Geometry: final body of the model. Coordinates: model frame, mm. A direction names the side the tool comes from. Coordinates: 2 decimals unless noted, no trailing zeros. Write each loop counter-clockwise with the first axis right and the second up, starting at its lowest first coordinate (ties: lowest second). Pieces come first, ordered by that corner, then holes. Notation, with made-up numbers: (88, -33) -> (127, -33) arc R11 cw to (127, -18) -> close; hole circle Ø7 at (82.25, 53). An arc over 180 degrees is marked (long way). One line per item, written item: value.
Autodesk Inventor part; units mm, degrees
ref_plane "YZ Plane" through (0, 0, 0) normal (1, 0, 0) x (0, 1, 0)
ref_plane "XZ Plane" through (0, 0, 0) normal (0, 1, 0) x (-1, 0, 0)
ref_plane "XY Plane" through (0, 0, 0) normal (0, 0, 1) x (1, 0, 0)
sketch "Boceto1" plane through (0, 0, 0) normal (1, 0, 0) x (0, 1, 0)
  line L0 (0, 0) -> (0, 14.3) construction
  line L1 (0, 14.3) -> (-23.8, 14.3) construction
  line L2 (-23.8, 14.3) -> (-23.8, 38.1) construction
  line L3 (-23.8, 38.1) -> (0, 14.3)
  circle A0 centre (0, 14.3) radius 14.3 construction
  line L4 (-10.1116, 4.1884) -> (-23.8, 17.8767)
  arc A1 (-10.1116, 4.1884) -> (0, 0) centre (0, 14.3) ccw
  line L5 (23.8, 38.1) -> (0, 14.3)
  line L6 (10.1116, 4.1884) -> (23.8, 17.8767)
  arc A2 (0, 0) -> (10.1116, 4.1884) centre (0, 14.3) ccw
  line L7 (23.8, 38.1) -> (23.8, 17.8767)
  circle A3 centre (-23.8, 38.1) radius 14.3 construction
  line L8 (-23.8, 38.1) -> (-23.8, 138.1)
  line L9 (-23.8, 17.8767) -> (-33.9116, 27.9884)
  line L10 (-38.1, 38.1) -> (-38.1, 138.1)
  line L11 (-38.1, 138.1) -> (-23.8, 138.1)
  arc A4 (-38.1, 38.1) -> (-33.9116, 27.9884) centre (-23.8, 38.1) ccw
  dimension "d0" = 14.3
  dimension "d1" = 23.8
  dimension "d2" = 23.8
  dimension "d3" = 28.6
  dimension "d4" = 100
  dimension "d7" = 23.8
  dimension "d8" = 47.6
  dimension "d9" = 47.9583
extrude "Extrusión1" add sketch "Boceto1" along normal mid plane 31.8
sketch "Boceto2" plane through (-15.9, -38.1, 138.1) normal (0, 0, 1) x (1, 0, 0)
  line L0 (0, 14.3) -> (31.8, 14.3) construction
  line L1 (31.8, 0) -> (31.8, 4.1884) construction
  line L2 (0, 14.3) -> (31.8, 0) construction
  line L3 (15.9, 7.15) -> (-3.1, 7.15) construction
  line L4 (-3.1, 7.15) -> (-3.1, 77.15) construction
  line L5 (-3.1, 77.15) -> (15.9, 77.15) construction
  line L6 (15.9, 77.15) -> (15.9, 7.15) construction
  line L7 (15.9, 7.15) -> (-54.1, 7.15) construction
  line L8 (-54.1, 7.15) -> (-54.1, 26.15) construction
  line L9 (-54.1, 26.15) -> (15.9, 26.15) construction
  line L10 (15.9, 26.15) -> (15.9, 7.15) construction
  circle A0 centre (15.9, 7.15) radius 30 construction
  line L11 (15.9, 77.15) -> (-3.1, 77.15)
  line L12 (-3.1, 30.3664) -> (-3.1, 77.15)
  line L13 (-54.1, 7.15) -> (-54.1, 26.15)
  line L14 (-54.1, 26.15) -> (-7.3164, 26.15)
  arc A1 (-3.1, 30.3664) -> (-7.3164, 26.15) centre (15.9, 7.15) ccw
  line L15 (-54.1, -11.85) -> (-54.1, 7.15) construction
  line L16 (15.9, -11.85) -> (-54.1, -11.85) construction
  line L17 (-7.3164, -11.85) -> (-54.1, -11.85)
  line L18 (-54.1, 7.15) -> (-54.1, -11.85)
  line L19 (15.9, -62.85) -> (-3.1, -62.85) construction
  line L20 (15.9, -62.85) -> (-3.1, -62.85)
  line L21 (-3.1, -62.85) -> (-3.1, 7.15) construction
  line L22 (-3.1, -62.85) -> (-3.1, -16.0664)
  arc A2 (-7.3164, -11.85) -> (-3.1, -16.0664) centre (15.9, 7.15) ccw
  line L23 (34.9, -62.85) -> (15.9, -62.85) construction
  line L24 (34.9, 7.15) -> (34.9, -62.85) construction
  line L25 (34.9, -16.0664) -> (34.9, -62.85)
  line L26 (15.9, -62.85) -> (34.9, -62.85)
  line L27 (85.9, 7.15) -> (85.9, -11.85) construction
  line L28 (85.9, 7.15) -> (85.9, -11.85)
  line L29 (85.9, -11.85) -> (15.9, -11.85) construction
  line L30 (85.9, -11.85) -> (39.1164, -11.85)
  arc A3 (34.9, -16.0664) -> (39.1164, -11.85) centre (15.9, 7.15) ccw
  line L31 (85.9, 26.15) -> (85.9, 7.15) construction
  line L32 (15.9, 26.15) -> (85.9, 26.15) construction
  line L33 (39.1164, 26.15) -> (85.9, 26.15)
  line L34 (85.9, 7.15) -> (85.9, 26.15)
  line L35 (15.9, 77.15) -> (34.9, 77.15) construction
  line L36 (15.9, 77.15) -> (34.9, 77.15)
  line L37 (34.9, 77.15) -> (34.9, 7.15) construction
  line L38 (34.9, 77.15) -> (34.9, 30.3664)
  arc A4 (39.1164, 26.15) -> (34.9, 30.3664) centre (15.9, 7.15) ccw
  point P0 (15.9, 38.1)
  point P1 (-54.1, 7.15)
  point P2 (85.9, 7.15)
  dimension "d10" = 19
  dimension "d11" = 70
  dimension "d12" = 70
  dimension "d13" = 19
  dimension "d14" = 60
  dimension "d17" = 360
extrude "Extrusión2" add sketch "Boceto2" along normal blind 5
sketch "Boceto3" plane through (-15.9, -38.1, 143.1) normal (0, 0, 1) x (1, 0, 0)
  arc A0 (39.1164, 26.15) -> (34.9, 30.3664) centre (15.9, 7.15) ccw
  circle A1 centre (15.9, 7.15) radius 7.9
  point P0 (15.9, 38.1)
  dimension "d21" = 15.8
extrude "Extrusión3" add sketch "Boceto3" along normal blind 15.8
sketch "Boceto4" plane through (0, -30.95, 158.9) normal (0, 0, 1) x (1, 0, 0)
  line L0 (12.7, 11.9) -> (-12.7, 11.9)
  line L1 (-12.7, 11.9) -> (-12.7, -11.9)
  line L2 (-12.7, -11.9) -> (12.7, -11.9)
  line L3 (12.7, -11.9) -> (12.7, 11.9)
  circle A0 centre (0, 0) radius 7.9
  point P0 (0, 30.95)
  point P1 (12.7, 0)
  point P2 (0, -11.9)
  dimension "d24" = 25.4
  dimension "d25" = 23.8
extrude "Extrusión4" add sketch "Boceto4" along normal blind 82.5 contours L3 L2 L1 L0 | A0
(1) Reachability of faces 4 (the flat face through (15.9, -26, 59)), 5 (the flat face through (-6, -25, 158.9)), 6 (the flat face through (19, -77, 141)), 7 (the flat face through (-0.2, -12.1, 26.4)), 8 (the flat face through (-12.7, -31, 200)) from +Z, -Z, +X, -X, +Y, -Y: full face, straight path, thin tool, end or side. Return the list, or none.
Responses:
face 4: -Z, +X, +Y, -Y
face 5: none
face 6: +Z, -Z, +X, -Y
face 7: +X, -X
face 8: +Z, -X, +Y, -Y
(2) Section C-C (y = -73.5). Return the cut outline in (x, z).
Responses:
outline: (-19, 138.1) -> (19, 138.1) -> (19, 143.1) -> (-19, 143.1) -> close
(3) First-contact query: pin 1 (19 mm diameter, centred on x = 2.5, y = -26, fed in from -Z); pin 2 (7 mm diameter, centred on y = -34.5, z = 199, fed in from -X); pin 3 (4 mm diameter, centred on y = -73, z = 141.5, fed in from -X). Flat tips, straight axial feed; report the tip coordinate or a pass-through.
Responses:
pin 1: stops at z = 10.58
pin 2: stops at x = -12.7
pin 3: stops at x = -19
(4) Pull-direction query (Z, two-part tool) for faces 1 (the cylindrical face through (-1.028, -38.783, 150.889)), 2 (the flat face through (19, 16, 141)), 3 (the flat face through (-0.223, 16.86, 10.937)); classes: released by +Z, released by -Z, zero draft, split by the parting line, or undercut.
Responses:
face 1: undercut
face 2: zero draft
face 3: released by -Z
(5) Section D-D (z = 62.5). Return the cut outline in (x, y).
Responses:
outline: (-15.9, -38.1) -> (15.9, -38.1) -> (15.9, -23.8) -> (-15.9, -23.8) -> close
(6) Section B-B (x = 0). Return the cut outline in (y, z).
Responses:
outline: (-100.95, 138.1) -> (-38.1, 138.1) -> (-38.1, 38.1) arc R14.3 ccw to (-33.91, 27.99) -> (-23.8, 17.88) -> (-10.11, 4.19) arc R14.3 ccw to (0, 0) arc R14.3 ccw to (10.11, 4.19) -> (23.8, 17.88) -> (23.8, 38.1) -> (0, 14.3) -> (-23.8, 38.1) -> (-23.8, 138.1) -> (39.05, 138.1) -> (39.05, 143.1) -> (-23.05, 143.1) -> (-23.05, 158.9) -> (-19.05, 158.9) -> (-19.05, 241.4) -> (-42.85, 241.4) -> (-42.85, 158.9) -> (-38.85, 158.9) -> (-38.85, 143.1) -> (-100.95, 143.1) -> close
(7) Line query: line 1 (Z direction, x = -3.5, y = -40); line 2 (Z direction, x = -11, y = -52.5); line 3 (Y direction, x = 6, z = 127.5). Output: solid intervals per line, ascending. Write a range as [from, to].
Responses:
line 1: z = [138.1, 143.1], [158.9, 241.4]
line 2: z = [138.1, 143.1]
line 3: y = [-38.1, -23.8]
(8) Section A-A (z = 23). Return the cut outline in (x, y).
Responses:
outline: (-15.9, -28.92) -> (15.9, -28.92) -> (15.9, -8.7) -> (-15.9, -8.7) -> close; (-15.9, 8.7) -> (15.9, 8.7) -> (15.9, 23.8) -> (-15.9, 23.8) -> close
